```python
from build123d import *

# Parameters (mm, degrees)
SKETCH1_R            = 2.4892
BOSS_EXTRUDE1_DEPTH  = 3.175
TRIGGER_CUTOUT_DEPTH = 3.175
SERVO_CUTOUT_DEPTH   = 3.175


with BuildPart() as part:
    # Sketch1 → Boss-Extrude1 (new body)
    with BuildSketch(Plane(origin=(0, 0, 0), x_dir=(1, 0, 0), z_dir=(0, 1, 0))):
        with BuildLine():
            Line((-6.8229868, -7.488197853), (47.14701474, -37.472309865))
            ThreePointArc((47.14701474, -37.472309865), (49.553689318, -38.298669515), (52.097667916, -38.242761734))
            Line((52.097667916, -38.242761734), (136.359344262, -21.308190288))
            ThreePointArc((136.359344262, -21.308190288), (139.866879533, -19.510833837), (141.916296901, -16.144354617))
            Line((141.916296901, -16.144354617), (166.90343399, 73.568749369))
            ThreePointArc((166.90343399, 73.568749369), (165.462253091, 80.188248266), (159.182077212, 82.728751949))
            Line((159.182077212, 82.728751949), (-4.366145722, 66.053653766))
            ThreePointArc((-4.366145722, 66.053653766), (-9.125920254, 63.663982971), (-10.969503308, 58.667265887))
            Line((-10.969503308, 58.667265887), (-10.288924124, -1.672992978))
            ThreePointArc((-10.288924124, -1.672992978), (-9.33910622, -5.047363397), (-6.8229868, -7.488197853))
        make_face()
        with Locations(Location((159.917634832, 75.514453101, 0), (0, 0, 270))):
            Circle(SKETCH1_R, mode=Mode.SUBTRACT)
        with Locations(Location((134.930497743, -14.198650885, 0), (0, 0, 270))):
            Circle(SKETCH1_R, mode=Mode.SUBTRACT)
        with Locations(Location((50.668821397, -31.133222331, 0), (0, 0, 270))):
            Circle(SKETCH1_R, mode=Mode.SUBTRACT)
        with Locations(Location((-3.719648143, 58.830829265, 0), (0, 0, 270))):
            Circle(SKETCH1_R, mode=Mode.SUBTRACT)
        with Locations(Location((-3.508126319, -0.086017173, 0), (0, 0, 270))):
            Circle(SKETCH1_R, mode=Mode.SUBTRACT)
    extrude(amount=BOSS_EXTRUDE1_DEPTH)

    # Sketch3 → trigger cutout (cut)
    with BuildSketch(Plane(origin=(0, 3.175, 0), x_dir=(1, 0, 0), z_dir=(0, 1, 0))):
        Polygon((41.255934536, -15.678441329), (66.468104622, -13.883980824), (70.774809833, -3.296663849), (70.032795293, 7.128640439), (58.56546888, 6.312460623), (53.862019579, 3.583115238), (41.255934536, 0), align=None)
    extrude(amount=-TRIGGER_CUTOUT_DEPTH, mode=Mode.SUBTRACT)

    # Sketch4 → servo cutout (cut)
    with BuildSketch(Plane(origin=(0, 3.175, 0), x_dir=(1, 0, 0), z_dir=(0, 1, 0))):
        with BuildLine():
            Line((69.425949058, 31.19523761), (94.572562087, 30.850872889))
            ThreePointArc((94.572562087, 30.850872889), (99.186221889, 26.850324024), (95.185673024, 22.236664221))
            Line((95.185673024, 22.236664221), (70.3413237, 18.334223888))
            ThreePointArc((70.3413237, 18.334223888), (69.247473844, 18.162406798), (68.140315886, 18.177568527))
            Line((68.140315886, 18.177568527), (42.993702858, 18.521933248))
            ThreePointArc((42.993702858, 18.521933248), (38.380043055, 22.522482114), (42.380591921, 27.136141916))
            Line((42.380591921, 27.136141916), (67.224941244, 31.03858225))
            ThreePointArc((67.224941244, 31.03858225), (68.318791101, 31.210399339), (69.425949058, 31.19523761))
        make_face()
    extrude(amount=-SERVO_CUTOUT_DEPTH, mode=Mode.SUBTRACT)


solid = part.part
```
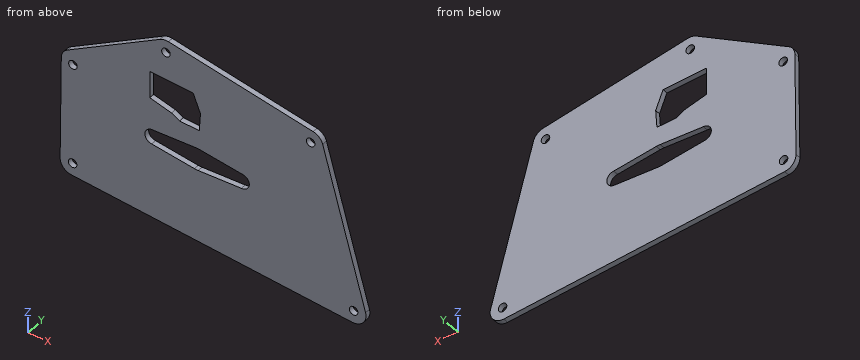
For this review, take the finished solid that the model builds, in its own axes (mm). Coordinates: 2 decimals unless noted, no trailing zeros. Write each loop counter-clockwise with the first axis right and the second up, starting at its lowest first coordinate (ties: lowest second). Pieces come first, ordered by that corner, then holes. Notation, with made-up numbers: (85, 30) - (115, 30) arc R24 ccw to (115, 63) - close; hole circle Ø9 at (-21.5, 72). An arc over 180 degrees is marked (long way). Answer in a Markdown table with one row per item. Add a question column.
Q1. We need section C-C, the plane z = -70. State the section outline as (x, y) points (3 decimals).
Q2. For P1, Ø1, axis at y = 1.5, z = 7.5, coming from the +X side; P2, Ø8, axis at x = 69.5, z = -50.5, coming from the -Y side, all flat-tipped, find the tip position at first contact; note any pin that passes through.
Q3. We need section A-A, the plane x = 89.5. State the section outline as (y, z) points (3 decimals).
Q4. For probe 1 along Z at (x, y) = (64.5, 2.55); probe 2 along Z at (x, y) = (45.5, 1); probe 3 along Z at (x, y) = (51.5, 1.15), list the stretches that pass through material, from the lowest coordinate up.
Q5. We need section D-D, the plane x = 108. State the section outline as (y, z) points (3 decimals).
Q6. We need section B-B, the plane y = 0.75. Count the separate pieces of the cut face and the enclosed holes in it, and give its area (3 significant figures).
Answer list:
| question | item | result |
|---|---|---|
| 1 | outline | (34.339, 0) - (165.909, 0) - (165.909, 3.175) - (34.339, 3.175) - close |
| 2 | P1 | stops at x = 144.46 |
| 2 | P2 | stops at y = 0 |
| 3 | outline | (0, -75.624) - (3.175, -75.624) - (3.175, -30.92) - (0, -30.92) - close; (0, -21.344) - (3.175, -21.344) - (3.175, 30.726) - (0, 30.726) - close |
| 4 | probe 1 | z = -73.08 to -30.61, -18.23 to -6.73, 14.02 to 35.75 |
| 4 | probe 2 | z = -71.14 to -27.63, -18.49 to -1.21, 15.38 to 36.56 |
| 4 | probe 3 | z = -71.75 to -28.57, -18.41 to -2.91, 14.95 to 28.79, 33.48 to 38.34 |
| 5 | outline | (0, -77.51) - (3.175, -77.51) - (3.175, 27.008) - (0, 27.008) - close |
| 6 | separate pieces | 1 |
| 6 | enclosed holes | 7 |
| 6 | area | 15,300 mm2 |
